Here's how the part is built. I have some questions about the finished solid (model axes, mm). A direction names the side the tool comes from. Coordinates: 2 decimals unless noted, no trailing zeros. Order: outer loops, then holes, each group sorted by start corner. A loop starts at its lowest first (then second) coordinate and runs counter-clockwise, first axis right, second up. Notation, with made-up numbers: M 11.25,-39.5 L 15.25,-39.5 A29 ccw 15.25,-1.5 Z; hole C 51,32 d4. An arc over 180 degrees is marked long. Answer as CSV lines item,"result". Start each with the question number.
```python
from build123d import *

# Parameters (mm, degrees)
SKETCH1_W           = 46.5
SKETCH1_H           = 24
BOSS_EXTRUDE1_DEPTH = 21
SHELL1_T            = -1.25
SKETCH2_W           = 19.75
SKETCH2_H           = 14.5
CUT_EXTRUDE1_DEPTH  = 57.384838388
SKETCH4_W           = 6.75
SKETCH4_H           = 6.5
SKETCH4_W_2         = 7.5
SKETCH4_H_2         = 17
CUT_EXTRUDE3_DEPTH  = 1.25
CUT_EXTRUDE4_REACH  = 57.358
SKETCH6_R           = 1.95
SKETCH7_W           = 10.375
SKETCH7_H           = 2.5
CUT_EXTRUDE5_DEPTH  = 1.25


with BuildPart() as part:
    # Sketch1 → Boss-Extrude1 (new body)
    with BuildSketch(Plane.XY):
        with Locations((22, 12)):
            Rectangle(SKETCH1_W, SKETCH1_H)
    extrude(amount=-BOSS_EXTRUDE1_DEPTH)

    # Shell1
    shell1_openings = [part.faces().sort_by_distance(p)[0] for p in [
        (22, 12, -21),
        (22, 24, -10.5),
    ]]
    offset(amount=SHELL1_T, openings=shell1_openings, kind=Kind.INTERSECTION)

    # Sketch2 → Cut-Extrude1 (cut, through all)
    with BuildSketch(Plane.ZY.offset(1.25)):
        with Locations((-11.125, 8.5)):
            Rectangle(SKETCH2_W, SKETCH2_H)
    extrude(amount=-CUT_EXTRUDE1_DEPTH, mode=Mode.SUBTRACT)

    # Sketch4 → Cut-Extrude3 (cut)
    with BuildSketch(Plane.XY):
        with Locations((8.375, 11.5)):
            Rectangle(SKETCH4_W, SKETCH4_H)
        with Locations((22.75, 15.75)):
            Rectangle(SKETCH4_W_2, SKETCH4_H_2)
    extrude(amount=-CUT_EXTRUDE3_DEPTH, mode=Mode.SUBTRACT)

    # Sketch6 → Cut-Extrude4 (cut, up to next)
    with BuildSketch(Plane(origin=(0, 0, 0), x_dir=(-1, 0, 0), z_dir=(0, -1, 0)), mode=Mode.PRIVATE) as cut_extrude4_sk1:
        with Locations(Location((-6.125, 9, 0), (0, 0, 90))):
            Circle(SKETCH6_R)
    cut_extrude4_tool1 = extrude(cut_extrude4_sk1.sketch, amount=-CUT_EXTRUDE4_REACH, mode=Mode.PRIVATE) & part.part
    # Sketch6 → Cut-Extrude4 (cut, up to next)
    with BuildSketch(Plane(origin=(0, 0, 0), x_dir=(-1, 0, 0), z_dir=(0, -1, 0)), mode=Mode.PRIVATE) as cut_extrude4_sk2:
        with Locations(Location((-37.875, 9, 0), (0, 0, 90))):
            Circle(SKETCH6_R)
    cut_extrude4_tool2 = extrude(cut_extrude4_sk2.sketch, amount=-CUT_EXTRUDE4_REACH, mode=Mode.PRIVATE) & part.part
    add(cut_extrude4_tool1.solids().sort_by_distance((6.125, 0, -9))[0], mode=Mode.SUBTRACT)
    add(cut_extrude4_tool2.solids().sort_by_distance((37.875, 0, -9))[0], mode=Mode.SUBTRACT)

    # Sketch7 → Cut-Extrude5 (cut)
    with BuildSketch(Plane.XY):
        with Locations((40.0625, 2.5)):
            Rectangle(SKETCH7_W, SKETCH7_H)
        with Locations((3.9375, 2.5)):
            Rectangle(SKETCH7_W, SKETCH7_H)
    extrude(amount=-CUT_EXTRUDE5_DEPTH, mode=Mode.SUBTRACT)


solid = part.part
```
1) Suppose I cut it at C-C on x = 41.5. Please give me the cut outline in (y, z), plus the area to 3 significant figures.
2) Suppose I cut it at A-A on y = 10.75. Please give me the cut outline in (x, z).
3) I need wall thicknesses on line 1 (X direction, y = 0.4, z = -9) (3 decimals); line 2 (X direction, y = 21, z = -8.75); line 3 (Y direction, x = 43.5, z = -6). Which ranges of each line are inside material? Lowest first, please. Write a range as [from, to].
4) Will these pins go through, and if not, where does the flat tip stop? pin 1 Ø1.4 at (x, z) = (-1, -6.5) entering from -Y; pin 2 Ø1 at (y, z) = (13.5, -16.5) entering from -X; pin 3 Ø1 at (x, y) = (24.5, 6.5) entering from -Z; pin 4 Ø0.6 at (x, z) = (22, -0.5) entering from +Y.
5) If we mould it in two halves opening along X, with no side actions, what happens to faces 6 (the face through (44, 20, -11)), 7 (the face through (-1.25, 18, -10)), 8 (the face through (22, 1.25, -10)), 9 (the face through (8, 8.25, -1))? For each: released by +X, released by -X, zero draft, split by the parting line, or undercut.
6) Suppose I cut it at D-D on z = -9. Please give me the cut outline in (x, y) (3 decimals).
7) Which directions (+Z, -Z, +X, -X, +Y, -Y) give clear straight access to the entire face, cutting with the end or side of a thin tool? Please do faces 1 (the face through (0, 20, -11)), 2 (the face through (-0.2, 24, -5.8)), 3 (the face through (19, 16, -1)), 4 (the face through (4, 3.75, -1)), 5 (the face through (5, 11, -1)).
8) Suppose I cut it at B-B on z = -3.5. Please give me the cut outline in (x, y), plus the area to 4 significant figures.
Output:
1,outline,"M 0,-21 L 1.25,-21 L 1.25,0 L 0,0 Z; M 3.75,-1.25 L 24,-1.25 L 24,0 L 3.75,0 Z"
1,area,"51.6 mm²"
2,outline,"M -1.25,-1.25 L 5,-1.25 L 5,0 L -1.25,0 Z; M 11.75,-1.25 L 19,-1.25 L 19,0 L 11.75,0 Z; M 26.5,-1.25 L 45.25,-1.25 L 45.25,0 L 26.5,0 Z"
3,line 1,"[-1.25, 4.175], [8.075, 35.925], [39.825, 45.25]"
3,line 2,"[-1.25, 0], [44, 45.25]"
3,line 3,"[0, 1.25]"
4,pin 1,"y = 0"
4,pin 2,"through"
4,pin 3,"z = -1.25"
4,pin 4,"y = 7.25"
5,face 6,"undercut"
5,face 7,"released by -X"
5,face 8,"zero draft"
5,face 9,"undercut"
6,outline,"M -1.25,0 L 4.175,0 L 4.175,1.25 L -1.25,1.25 Z; M -1.25,15.75 L 0,15.75 L 0,24 L -1.25,24 Z; M 8.075,0 L 35.925,0 L 35.925,1.25 L 8.075,1.25 Z; M 39.825,0 L 45.25,0 L 45.25,1.25 L 39.825,1.25 Z; M 44,15.75 L 45.25,15.75 L 45.25,24 L 44,24 Z"
7,face 1,"-Z, +Y"
7,face 2,"+Z, -Z, +X, -X, +Y"
7,face 3,"+Z, -Z, +Y"
7,face 4,"+Z, -Z, -X"
7,face 5,"+Z, -Z"
8,outline,"M -1.25,0 L 45.25,0 L 45.25,1.25 L -1.25,1.25 Z; M -1.25,15.75 L 0,15.75 L 0,24 L -1.25,24 Z; M 44,15.75 L 45.25,15.75 L 45.25,24 L 44,24 Z"
8,area,"78.75 mm²"
